from build123d import *

# Parameters (mm, degrees)
SKETCH_R           = 12.7
SKETCH_R_2         = 8.7
PAD_DEPTH          = 20
PAD001_DEPTH       = 3.34
POLARPATTERN_COUNT = 2


with BuildPart() as part:
    # Sketch → Pad (new body)
    with BuildSketch(Plane.XY):
        Circle(SKETCH_R)
        Circle(SKETCH_R_2, mode=Mode.SUBTRACT)
    extrude(amount=PAD_DEPTH)

    # Sketch001 (on Face4 of Pad) → Pad001 (join)
    with BuildSketch(Plane.XY.offset(20)):
        with BuildLine():
            ThreePointArc((3.5, 12.208194), (0, 12.7), (-3.5, 12.208194))
            Line((-2.681395, 13.435033), (-3.5, 12.208194))
            ThreePointArc((2.681395, 13.435033), (0, 13.7), (-2.681395, 13.435033))
            Line((2.681395, 13.435033), (3.5, 12.208194))
        make_face()
    pad001 = extrude(amount=-PAD001_DEPTH)

    # PolarPattern: Pad001 ×2 about axis
    polarpattern_axis = Axis((0, 0, 20), (0, 0, 1))
    for i in range(1, POLARPATTERN_COUNT):
        add(pad001.rotate(polarpattern_axis, i * 360 / POLARPATTERN_COUNT))


solid = part.part
Build history of the part. All positions in model axes, mm. A direction names the side the tool comes from. Coordinates: 2 decimals unless noted, no trailing zeros. Order: outer loops, then holes, each group sorted by start corner. A loop starts at its lowest first (then second) coordinate and runs counter-clockwise, first axis right, second up. Notation, with made-up numbers: (59.25, 10.5) - (105.25, 10.5) arc R24 cw to (105.25, 41.5) - close; hole circle Ø6 at (43, 51). An arc over 180 degrees is marked (long way). Put each result on its own line as item: value.
1. Saw through at D-D (y = 5.75). Write the cut outline in (x, z).
Answer sheet:
outline: (-11.32, 0) - (-6.53, 0) - (-6.53, 20) - (-11.32, 20) - close; (6.53, 0) - (11.32, 0) - (11.32, 20) - (6.53, 20) - close
2. Saw through at B-B (y = 0). Write the cut outline in (x, z), and give its area (3 significant figures).
Answer sheet:
outline: (-12.7, 0) - (-8.7, 0) - (-8.7, 20) - (-12.7, 20) - close; (8.7, 0) - (12.7, 0) - (12.7, 20) - (8.7, 20) - close
area: 160 mm^2
3. Saw through at C-C (z = 17). Write the cut outline in (x, y).
Answer sheet:
outline: (-3.5, -12.21) - (-2.68, -13.44) arc R13.7 ccw to (2.68, -13.44) - (3.5, -12.21) arc R12.7 ccw to (3.5, 12.21) - (2.68, 13.44) arc R13.7 ccw to (-2.68, 13.44) - (-3.5, 12.21) arc R12.7 ccw to start; hole circle Ø17.4 at (0, 0)
4. Probe line 1 along Y through (x, z) = (0, 4.5); line 2 along Y through (x, z) = (-3, 9.75); line 3 along X through (y, z) = (5.5, 12). List the from-to ranges inside material, lowest first. Write a range as [from, to].
Answer sheet:
line 1: y = [-12.7, -8.7], [8.7, 12.7]
line 2: y = [-12.34, -8.17], [8.17, 12.34]
line 3: x = [-11.45, -6.74], [6.74, 11.45]
5. Pull direction Y, two halves, no side cores. Call faces 1 (the face through (-1.886, -8.493, 9.86)), 2 (the face through (3.085, 12.83, 18.353)), 3 (the face through (0, 13, 16.66)), 4 (the face through (0, -13.7, 18.4)): pulls with the +Y half, pulls with the -Y half, needs draft (parallel to the pull), parting line crosses it, or undercut.
Answer sheet:
face 1: undercut
face 2: pulls with the +Y half
face 3: needs draft
face 4: pulls with the -Y half
6. Tool access for faces 5 (the face through (-3.085, -12.83, 18.353)), 6 (the face through (12.114, 3.815, 9.86)): list every direction of +Z, -Z, +X, -X, +Y, -Y with a clear straight run to the whole face (end or side of a thin tool).
Answer sheet:
face 5: +Z, -Z, -X, -Y
face 6: -Z
7. Drop flat-ended pins along their axis: P1, Ø3, axis at x = -8, z = 6, coming from the +Y side; P2, Ø1.5, axis at x = 9, z = 17.5, coming from the +Y side; P3, Ø3, axis at x = 4, z = 9.5, coming from the -Y side. Give the stop position or say it passes through.
Answer sheet:
P1: stops at y = 10.91
P2: stops at y = 9.66
P3: stops at y = -12.45
8. Saw through at A-A (x = 0). Write the cut outline in (y, z), and give its area (3 significant figures).
Answer sheet:
outline: (-13.7, 16.66) - (-12.7, 16.66) - (-12.7, 0) - (-8.7, 0) - (-8.7, 20) - (-13.7, 20) - close; (8.7, 0) - (12.7, 0) - (12.7, 16.66) - (13.7, 16.66) - (13.7, 20) - (8.7, 20) - close
area: 167 mm^2
